```python
from build123d import *

# Parameters (mm, degrees)
CROQUIS3_R            = 1
CORTAR_EXTRUIR1_DEPTH = 3


with BuildPart() as part:
    # Croquis2 → Revolución1 (revolve)
    with BuildSketch(Plane(origin=(0, 0, 0), x_dir=(0, 0, -1), z_dir=(1, 0, 0))):
        Polygon((0, 1.5), (0, 3), (1.5, 3), (1.5, 3.5), (-0.5, 3.5), (-0.5, 4.5), (1, 4.5), (1, 10.5), (-1, 10.5), (-1, 4.5), (-4, 4.5), (-4, 3), (-1.525538697, 3), (-1.525538697, 1.5), align=None)
    revolve(axis=Axis((0, 0, 0), (0, 0, 1)))

    # Croquis3 → Cortar-Extruir1 (cut)
    with BuildSketch(Plane(origin=(0, 0, -1), x_dir=(-1, 0, 0), z_dir=(0, 0, -1))):
        with Locations((7.5, 2.5)):
            Circle(CROQUIS3_R)
        with Locations((0, 7.5)):
            Circle(CROQUIS3_R)
        with Locations((7.5, 0)):
            Circle(CROQUIS3_R)
        with Locations((-7.5, 0)):
            Circle(CROQUIS3_R)
        with Locations((0, -7.5)):
            Circle(CROQUIS3_R)
        with Locations((2.5, -7.5)):
            Circle(CROQUIS3_R)
        with Locations((-7.5, -2.5)):
            Circle(CROQUIS3_R)
        with Locations((-2.5, 7.5)):
            Circle(CROQUIS3_R)
        with Locations((7.5, -2.5)):
            Circle(CROQUIS3_R)
        with Locations((-2.5, -7.5)):
            Circle(CROQUIS3_R)
        with Locations((-7.5, 2.5)):
            Circle(CROQUIS3_R)
        with Locations((2.5, 7.5)):
            Circle(CROQUIS3_R)
    extrude(amount=-CORTAR_EXTRUIR1_DEPTH, mode=Mode.SUBTRACT)


solid = part.part
```
Input: part model. Units: mm. Frame: model coordinates. A direction names the side the tool comes from. Round coordinates to 2 decimals unless told otherwise and drop trailing zeros. Write each loop counter-clockwise with the first axis right and the second up, starting at its lowest first coordinate (ties: lowest second). Pieces come first, ordered by that corner, then holes. Notation, with made-up numbers: (84.5, 9) - (121.5, 9) arc R18 ccw to (121.5, 33) - close; hole circle Ø5 at (43.5, 86). An arc over 180 degrees is marked (long way). Write item = value, one per line.
(1) Pull-direction query (X, two-part tool) for faces 4 (the flat face through (0, -5, -1)), 5 (the cylindrical face through (-2.37, 8.49, -0.01)), 6 (the cylindrical face through (-3.2, 10, 0)); classes: +X half, -X half, draft (parallel to the pull), parting line (faces both ways), or undercut.
Geometry check:
face_4 = draft
face_5 = undercut
face_6 = parting line
(2) Section query D-D on x = -1.25. Output: boundary loops of the cut face in (y, z), then the cut area to 3 significant figures.
Geometry check:
outline = (-10.43, -1) - (-4.32, -1) - (-4.32, 0.5) - (-3.27, 0.5) - (-3.27, -1.5) - (-2.73, -1.5) - (-2.73, 0) - (-0.83, 0) - (-0.83, 1.53) - (-2.73, 1.53) - (-2.73, 4) - (-4.32, 4) - (-4.32, 1) - (-10.43, 1) - close; (0.83, 0) - (2.73, 0) - (2.73, -1.5) - (3.27, -1.5) - (3.27, 0.5) - (4.32, 0.5) - (4.32, -1) - (10.43, -1) - (10.43, 1) - (4.32, 1) - (4.32, 4) - (2.73, 4) - (2.73, 1.53) - (0.83, 1.53) - close
area = 43.5 mm^2
(3) Section query A-A on y = -2.25. State how many separate pieces and enclosed holes the cut face has, then the cut area to 3 significant figures.
Geometry check:
separate_pieces = 3
enclosed_holes = 0
area = 39.9 mm^2
(4) Section query C-C on y = 7.75. Output: boundary loops of the cut face in (x, z), then the cut area to 3 significant figures.
Geometry check:
outline = (-7.08, -1) - (-3.47, -1) - (-3.47, 1) - (-7.08, 1) - close; (-1.53, -1) - (-0.97, -1) - (-0.97, 1) - (-1.53, 1) - close; (0.97, -1) - (1.53, -1) - (1.53, 1) - (0.97, 1) - close; (3.47, -1) - (7.08, -1) - (7.08, 1) - (3.47, 1) - close
area = 16.7 mm^2
(5) Access query for faces 1 (the flat face through (3, 1, 4)), 2 (the cylindrical face through (-4.46, -0.59, -0.26)), 3 (the flat face through (1.3, 1.3, 1.526)). Directions: +Z, -Z, +X, -X, +Y, -Y. A direction counts if a zero-diameter tool reaches every point of the face in a straight line with its end or side. Return the directions, or none.
Geometry check:
face_1 = +Z, +X, -X, +Y, -Y
face_2 = -Z
face_3 = +Z
(6) Contact query for flat-ended pins moving along their axis: pin 1 Ø6.5 at (x, y) = (-1, 1) entering from +Z; pin 2 Ø2.5 at (x, y) = (-2.5, 7.5) entering from +Z; pin 3 Ø3 at (y, z) = (-6.5, 0) entering from -X; pin 4 Ø1 at (y, z) = (0, 3) entering from +X. Output: stop coordinate, or through.
Geometry check:
pin_1 = 4
pin_2 = 1
pin_3 = -9.23
pin_4 = 4.5
(7) Material intervals for probe 1 along Y at (x, z) = (0, -0.2); probe 2 along X at (y, z) = (0, -1.1); probe 3 along Y at (x, z) = (7.5, 0.45), sorted ascending.
Geometry check:
probe_1 = -10.5 to -8.5, -6.5 to -4.5, -3.5 to -3, 3 to 3.5, 4.5 to 6.5, 8.5 to 10.5
probe_2 = -3.5 to -3, 3 to 3.5
probe_3 = -7.35 to -3.5, -1.5 to -1, 1 to 1.5, 3.5 to 7.35
